Read the model definition and answer for the solid it produces. Units are mm, in the model's axes. Coordinates: 2 decimals unless noted, no trailing zeros. Write each loop counter-clockwise with the first axis right and the second up, starting at its lowest first coordinate (ties: lowest second). Pieces come first, ordered by that corner, then holes. Notation, with made-up numbers: (-24, 48) -> (21, 48) arc R14 cw to (21, 65) -> close; hole circle Ø8 at (-24.75, 50.25). An arc over 180 degrees is marked (long way). Return JSON: item names as keys, results as strings.
from build123d import *

# Parameters (mm, degrees)
F0_W     = 600
F0_H     = 100
F3_DEPTH = 50
F1_SIZE  = 49.99999
F4_SIZE  = 49.99999
F2_R     = 5


# Not quite as in the source:
# - a fillet or chamfer is up to 0.001 mm smaller than in the source, because OpenCascade refuses the exact size


with BuildPart() as f3:
    # F0 (on Front) → F3 (new body)
    with BuildSketch(Plane.XZ):
        with Locations((-350.3373948519, 50)):
            Rectangle(F0_W, F0_H)
    extrude(amount=F3_DEPTH)

    # F1 (size 50 in the source; OpenCascade refuses exactly that, so slightly less here)
    f1_edges = [f3.edges().sort_by_distance(p)[0] for p in [
        (-50.337395, -50, 50),
    ]]
    chamfer(f1_edges, length=F1_SIZE)

    # F4 (size 50 in the source; OpenCascade refuses exactly that, so slightly less here)
    f4_edges = [f3.edges().sort_by_distance(p)[0] for p in [
        (-650.337395, -50, 50),
    ]]
    chamfer(f4_edges, length=F4_SIZE)

    # F2
    f2_edges = [f3.edges().sort_by_distance(p)[0] for p in [
        (-350.337395, -50, 0),
        (-350.337395, -50, 100),
        (-350.337395, 0, 100),
        (-350.337395, 0, 0),
    ]]
    fillet(f2_edges, radius=F2_R)


solid = f3.part
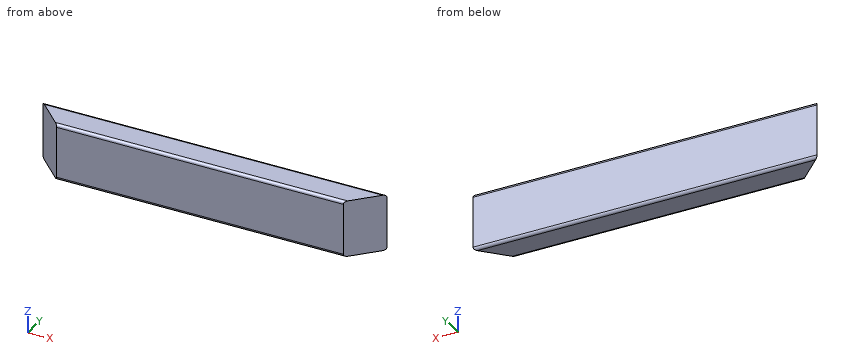
1. Flat-ended cylindrical pins translate along their axes: pin 1 Ø3 at (y, z) = (-9.5, 48) entering from -X; pin 2 Ø5 at (y, z) = (-27.5, 28) entering from +X; pin 3 Ø6 at (y, z) = (-8.5, 79) entering from +X. Find the tip coordinate at first contact, or state that the pin passes through.
Taken from the geometry:
{"pin 1": "stops at x = -642.34", "pin 2": "stops at x = -75.34", "pin 3": "stops at x = -55.84"}
2. The part is cut by section B-B (y = -39.5). Determine the outline of the cut face in (x, z), then the cut area to 3 significant figures.
Taken from the geometry:
{"outline": "(-610.84, 0) -> (-89.84, 0) -> (-89.84, 100) -> (-610.84, 100) -> close", "area": "52,100 mm2"}
3. The part is cut by section C-C (y = -15.5). Determine the outline of the cut face in (x, z), then the cut area to 3 significant figures.
Taken from the geometry:
{"outline": "(-634.84, 0) -> (-65.84, 0) -> (-65.84, 100) -> (-634.84, 100) -> close", "area": "56,900 mm2"}
4. Consider L1, parallel to X at y = -23, z = 40; L2, parallel to X at y = -46, z = 54; L3, parallel to Z at x = -273.5, y = -47. Determine where each line is inside the solid, lowest interval first.
Taken from the geometry:
{"L1": "x = -627.34 to -73.34", "L2": "x = -604.34 to -96.34", "L3": "z = 0.42 to 99.58"}
